The model under review builds one solid part; all positions refer to its coordinate system, in mm. Face numbers are marked on the shaded views. A direction names the side the tool comes from. Round coordinates to 2 decimals unless told otherwise and drop trailing zeros. Order: outer loops, then holes, each group sorted by start corner. A loop starts at its lowest first (then second) coordinate and runs counter-clockwise, first axis right, second up. Notation, with made-up numbers: (64.25, 55) - (82.25, 55) arc R18 cw to (82.25, 78) - close; hole circle Ø9 at (-11.5, -30). An arc over 180 degrees is marked (long way). One line per question, with ' | ' between items. Start each with the question number.
Item 1: Add section C-C on x = 9.25. State the section outline as (y, z) points (3 decimals), and give its area (3 significant figures).
Item 2: Add section A-A on z = -13. State the section outline as (x, y) points (3 decimals).
Item 3: Insertion check: pin 1 Ø12 at (y, z) = (3.5, -1) entering from -X; pin 2 Ø4 at (x, y) = (6.5, 4.5) entering from -Z; pin 3 Ø3.5 at (x, z) = (9.5, -11.5) entering from -Y; pin 4 Ø0.8 at (x, y) = (10, -0.5) entering from -Z. Each pin has a flat end and moves straight along its axis. Give the tip position at first contact, or say it passes through.
Item 4: Add section B-B on y = 4. State the section outline as (x, z) points, and give its area (3 significant figures).
Item 5: For L1, parallel to Z at x = -7, y = 8.5; L2, parallel to Y at x = -10.5, z = -4.5; L3, parallel to Y at x = -16, z = -11.25, list the stretches that pass through material, from the lowest coordinate up. Write a range as [from, to].
Item 6: Tool access review of the marked faces 5, 6, 7, 8 and 9: name each direction out of +Z, -Z, +X, -X, +Y, -Y from which nothing blocks a thin tool from reaching the whole face with its end or side.
Item 7: Add section D-D on z = -22. State the section outline as (x, y) points, and give its area (3 significant figures).
Item 8: Draft analysis for pull direction X (two halves, no side actions). For the marked faces 1, 2, 3 and 4, state which applies: +X half, -X half, draft (parallel to the pull), parting line (faces both ways), or undercut.
from build123d import *

# Parameters (mm, degrees)
F0_W           = 13.375
F0_H           = 2
F1_DEPTH       = 18.25
F2_R           = 1.7808687455
F2_R_2         = 1.7800904517
F3_DEPTH       = 2
F4_W           = 11.3
F4_H           = 30
F5_DEPTH       = 18.25
F6_W           = 26
F6_H           = 6.5
F7_DEPTH       = 30
F9_DEPTH       = 30
F11_DEPTH      = 13
F11_DEPTH_BACK = 13
F12_R          = 1.375
F13_DEPTH      = 4.8
F14_W          = 5.5
F14_H          = 5.5
F15_DEPTH      = 1.5
F16_T1_DEPTH   = 27.75
F16_T3_DEPTH   = 27.75
F16_T5_DEPTH   = 59
F17_SIZE2      = 10.3923048454
F17_SIZE       = 6
F18_T1_DEPTH   = 20.7323463904
F18_T3_DEPTH   = 6.4746360003
F18_T5_DEPTH   = 38.5573463904
F18_T7_DEPTH   = 1.5286731952
F18_T9_DEPTH   = 7.7786731952
F18_T11_DEPTH  = 6.4746360003
F18_T13_DEPTH  = 7.7786731952
F18_T18_DEPTH  = 4.8857735151
F18_T23_DEPTH  = 10.5573463904
F18_T29_DEPTH  = 4.8857735151
F18_T39_DEPTH  = 2.5573463904
F18_T43_DEPTH  = 8.8073463904
F18_T50_DEPTH  = 4.8857735151
F18_T54_DEPTH  = 10.5573463904
F18_T61_DEPTH  = 2.5573463904
F18_T65_DEPTH  = 8.8073463904
F18_T72_DEPTH  = 10.5573463904
F18_T76_DEPTH  = 4.8857735151


# Not quite as in the source:
# - a fillet or chamfer that OpenCascade refuses, or shapes differently, is made with other operations: its cross-section is extruded or revolved along the edge and cut away or added


with BuildPart() as f1:
    # F0 (on Right) → F1 (new body, symmetric)
    with BuildSketch(Plane.YZ):
        with Locations((6.6875, 1)):
            Rectangle(F0_W, F0_H)
    extrude(amount=F1_DEPTH, both=True)

    # F2 (on face) → F3 (cut, through all)
    with BuildSketch(Plane.XY.offset(2)):
        with Locations((6.5276143141, 4)):
            Circle(F2_R)
        with Locations((-6.3883271068, 4)):
            Circle(F2_R_2)
    extrude(amount=-F3_DEPTH, mode=Mode.SUBTRACT)

    # F4 (on Right) → F5 (join, symmetric)
    with BuildSketch(Plane.YZ):
        with Locations((-5.65, -13)):
            Rectangle(F4_W, F4_H)
    extrude(amount=F5_DEPTH, both=True)

    # F6 (on face) → F7 (cut, through all)
    with BuildSketch(Plane(origin=(0, 0, -28), x_dir=(1, 0, 0), z_dir=(0, 0, -1))):
        with Locations((0, 8.05)):
            Rectangle(F6_W, F6_H)
    extrude(amount=-F7_DEPTH, mode=Mode.SUBTRACT)

    # F8 (on face) → F9 (cut, through all)
    with BuildSketch(Plane(origin=(0, 0, -28), x_dir=(1, 0, 0), z_dir=(0, 0, -1))):
        Polygon((6.25, 4.8), (-6.25, 4.8), (-4.25, 2.8), (4.25, 2.8), align=None)
    extrude(amount=-F9_DEPTH, mode=Mode.SUBTRACT)

    # F10 (on Right) → F11 (cut, two sides)
    with BuildSketch(Plane.YZ) as f11_sk:
        Polygon((-4.8, -28), (-2.8, -28), (-4.8, -16), align=None)
    extrude(amount=F11_DEPTH, mode=Mode.SUBTRACT)
    extrude(f11_sk.sketch, amount=-F11_DEPTH_BACK, mode=Mode.SUBTRACT)

    # F12 (on face) → F13 (cut, through all)
    with BuildSketch(Plane.XZ.offset(4.8)):
        with Locations((-9.25, -13)):
            Circle(F12_R)
        with Locations((9.25, -13)):
            Circle(F12_R)
    extrude(amount=-F13_DEPTH, mode=Mode.SUBTRACT)

    # F14 (on face) → F15 (cut)
    with BuildSketch(Plane(origin=(0, 0, 0), x_dir=(-1, 0, 0), z_dir=(0, 1, 0))):
        with Locations((-9.25, -13)):
            Rectangle(F14_W, F14_H)
        with Locations((9.25, -13)):
            Rectangle(F14_W, F14_H)
    extrude(amount=-F15_DEPTH, mode=Mode.SUBTRACT)

    # F16: fillet of radius 4.5 on 3 edges, made by hand

    # F16_s2 → F16_t1 (cut)
    with BuildSketch(Plane.YZ.offset(-29.5)):
        with BuildLine():
            ThreePointArc((-11.3, -23.5), (-9.9819805153, -26.6819805153), (-6.8, -28))
            Line((-6.8, -28), (-11.3, -28))
            Line((-11.3, -28), (-11.3, -23.5))
        make_face()
    extrude(amount=F16_T1_DEPTH, mode=Mode.SUBTRACT)

    # F16_s4 → F16_t3 (cut)
    with BuildSketch(Plane.YZ.offset(1.75)):
        with BuildLine():
            ThreePointArc((-6.8, -28), (-9.9819805153, -26.6819805153), (-11.3, -23.5))
            Line((-11.3, -23.5), (-11.3, -28))
            Line((-11.3, -28), (-6.8, -28))
        make_face()
    extrude(amount=F16_T3_DEPTH, mode=Mode.SUBTRACT)

    # F16_s6 → F16_t5 (cut)
    with BuildSketch(Plane.YZ.offset(-29.5)):
        with BuildLine():
            ThreePointArc((-4.5, -28), (-1.3180194847, -26.6819805153), (0, -23.5))
            Line((0, -23.5), (0, -28))
            Line((0, -28), (-4.5, -28))
        make_face()
    extrude(amount=F16_T5_DEPTH, mode=Mode.SUBTRACT)

    # F17
    f17_edges = [f1.edges().sort_by_distance(p)[0] for p in [
        (-15.625, -11.3, 2),
        (15.625, -11.3, 2),
    ]]
    f17_side = f1.faces().sort_by_distance((-0.00209, 3.324537, 2))[0]
    chamfer(f17_edges, length=F17_SIZE, length2=F17_SIZE2, reference=f17_side)

    # F18: chamfer of 0.4 on 14 edges, made by hand

    # F18_s2 → F18_t1 (cut)
    with BuildSketch(Plane.XZ.offset(-14.4036731952)):
        Polygon((-18.25, 1.6), (-17.85, 2), (-18.25, 2), align=None)
        Polygon((17.85, 2), (18.25, 1.6), (18.25, 2), align=None)
    extrude(amount=F18_T1_DEPTH, mode=Mode.SUBTRACT)

    # F18_s4 → F18_t3 (cut)
    with BuildSketch(Plane.YZ.offset(-18.8623180002)):
        Polygon((-5.4154700538, 1.8), (-5.0690598923, 2), (-5.3, 2), align=None)
    extrude(amount=F18_T3_DEPTH, mode=Mode.SUBTRACT)

    # F18_s6 → F18_t5 (cut)
    with BuildSketch(Plane.YZ.offset(-19.2786731952)):
        Polygon((12.975, 2), (13.375, 1.6), (13.375, 2), align=None)
    extrude(amount=F18_T5_DEPTH, mode=Mode.SUBTRACT)

    # F18_s8 → F18_t7 (cut)
    with BuildSketch(Plane.XZ.offset(4.8)):
        Polygon((-13.4, 2), (-13, 1.6), (-13, 2), align=None)
        Polygon((13.4, 2), (13, 1.6), (13, 2), align=None)
    extrude(amount=F18_T7_DEPTH, mode=Mode.SUBTRACT)

    # F18_s10 → F18_t9 (cut)
    with BuildSketch(Plane.YZ.offset(-13)):
        Polygon((-4.4, 2), (-4.8, 1.6), (-4.8, 2), align=None)
    extrude(amount=F18_T9_DEPTH, mode=Mode.SUBTRACT)

    # F18_s12 → F18_t11 (cut)
    with BuildSketch(Plane.YZ.offset(12.3876819998)):
        Polygon((-5.0690598923, 2), (-5.4154700538, 1.8), (-5.3, 2), align=None)
    extrude(amount=F18_T11_DEPTH, mode=Mode.SUBTRACT)

    # F18_s14 → F18_t13 (cut)
    with BuildSketch(Plane.YZ.offset(5.2213268048)):
        Polygon((-4.4, 2), (-4.8, 1.6), (-4.8, 2), align=None)
    extrude(amount=F18_T13_DEPTH, mode=Mode.SUBTRACT)


with BuildPart() as f18_tool16:
    # F18_s17 → F18_t18 (new body)
    with BuildSketch(Plane(origin=(-6.2523817919, -6.2523817919, 0), x_dir=(0, 0, 1), z_dir=(0.7071067812, 0.7071067812, 0))):
        Polygon((2, -1.4253048327), (1.6, -1.0253048327), (2, -1.0253048327), align=None)
    extrude(amount=F18_T18_DEPTH)

    split(bisect_by=Plane.XZ.offset(2.8), keep=Keep.TOP)


with BuildPart() as f1_1:
    add(f1.part)

    # F18_t15: cut F18_tool16
    add(f18_tool16.part, mode=Mode.SUBTRACT)


with BuildPart() as f18_tool21:
    # F18_s22 → F18_t23 (new body)
    with BuildSketch(Plane.YZ.offset(-5.2786731952)):
        Polygon((-2.4, 2), (-2.8, 1.6), (-2.8, 2), align=None)
    extrude(amount=F18_T23_DEPTH)

    split(bisect_by=Plane(origin=(-0.725, 0.725, 0), x_dir=(0, 0, 1), z_dir=(0.7071067812, -0.7071067812, 0)), keep=Keep.TOP)

    split(bisect_by=Plane(origin=(0.725, 0.725, 0), x_dir=(0, 0, 1), z_dir=(-0.7071067812, -0.7071067812, 0)), keep=Keep.TOP)


with BuildPart() as f1_2:
    add(f1_1.part)

    # F18_t20: cut F18_tool21
    add(f18_tool21.part, mode=Mode.SUBTRACT)


with BuildPart() as f18_tool27:
    # F18_s28 → F18_t29 (new body)
    with BuildSketch(Plane(origin=(2.7976182081, -2.7976182081, 0), x_dir=(0, 0, 1), z_dir=(0.7071067812, -0.7071067812, 0))):
        Polygon((2, -1.4253048327), (1.6, -1.0253048327), (2, -1.0253048327), align=None)
    extrude(amount=F18_T29_DEPTH)

    split(bisect_by=Plane.XZ.offset(2.8), keep=Keep.TOP)


with BuildPart() as f1_3:
    add(f1_2.part)

    # F18_t26: cut F18_tool27
    add(f18_tool27.part, mode=Mode.SUBTRACT)

    # F18_s31 → F18_t32 (revolve, cut)
    with BuildSketch(Plane.XZ.offset(-4)):
        Polygon((-4.2082366551, 2), (-4.6082366551, 1.6), (-4.6082366551, 2), align=None)
    revolve(axis=Axis((-6.3883271068, 4, 2), (0, 0, 1)), mode=Mode.SUBTRACT)

    # F18_s33 → F18_t34 (revolve, cut)
    with BuildSketch(Plane.XZ.offset(-4)):
        Polygon((8.7084830596, 2), (8.3084830596, 1.6), (8.3084830596, 2), align=None)
    revolve(axis=Axis((6.5276143141, 4, 2), (0, 0, 1)), mode=Mode.SUBTRACT)


with BuildPart() as f18_tool37:
    # F18_s38 → F18_t39 (new body)
    with BuildSketch(Plane.XZ.offset(6.3286731952)):
        Polygon((-13.4, 2), (-13, 1.6), (-13, 2), align=None)
    extrude(amount=-F18_T39_DEPTH)

    split(bisect_by=Plane.XZ.offset(4.8), keep=Keep.BOTTOM)


with BuildPart() as f18_tool41:
    # F18_s42 → F18_t43 (new body)
    with BuildSketch(Plane.YZ.offset(-14.0286731952)):
        Polygon((-4.4, 2), (-4.8, 1.6), (-4.8, 2), align=None)
    extrude(amount=F18_T43_DEPTH)

    split(bisect_by=Plane.YZ.offset(-13), keep=Keep.BOTTOM)


with BuildPart() as f18_tool37_1:
    add(f18_tool37.part)

    # F18_t45: intersect F18_tool41
    add(f18_tool41.part, mode=Mode.INTERSECT)


with BuildPart() as f1_4:
    add(f1_3.part)

    # F18_t35: cut F18_tool37
    add(f18_tool37_1.part, mode=Mode.SUBTRACT)


with BuildPart() as f18_tool48:
    # F18_s49 → F18_t50 (new body)
    with BuildSketch(Plane(origin=(-6.2523817919, -6.2523817919, 0), x_dir=(0, 0, 1), z_dir=(0.7071067812, 0.7071067812, 0))):
        Polygon((2, -1.4253048327), (1.6, -1.0253048327), (2, -1.0253048327), align=None)
    extrude(amount=F18_T50_DEPTH)

    split(bisect_by=Plane.XZ.offset(2.8), keep=Keep.BOTTOM)


with BuildPart() as f18_tool52:
    # F18_s53 → F18_t54 (new body)
    with BuildSketch(Plane.YZ.offset(-5.2786731952)):
        Polygon((-2.4, 2), (-2.8, 1.6), (-2.8, 2), align=None)
    extrude(amount=F18_T54_DEPTH)

    split(bisect_by=Plane(origin=(-0.725, 0.725, 0), x_dir=(0, 0, 1), z_dir=(-0.7071067812, 0.7071067812, 0)), keep=Keep.TOP)


with BuildPart() as f18_tool48_1:
    add(f18_tool48.part)

    # F18_t56: intersect F18_tool52
    add(f18_tool52.part, mode=Mode.INTERSECT)


with BuildPart() as f1_5:
    add(f1_4.part)

    # F18_t46: cut F18_tool48
    add(f18_tool48_1.part, mode=Mode.SUBTRACT)


with BuildPart() as f18_tool59:
    # F18_s60 → F18_t61 (new body)
    with BuildSketch(Plane.XZ.offset(3.7713268048)):
        Polygon((13.4, 2), (13, 1.6), (13, 2), align=None)
    extrude(amount=F18_T61_DEPTH)

    split(bisect_by=Plane.XZ.offset(4.8), keep=Keep.BOTTOM)


with BuildPart() as f18_tool63:
    # F18_s64 → F18_t65 (new body)
    with BuildSketch(Plane.YZ.offset(5.2213268048)):
        Polygon((-4.4, 2), (-4.8, 1.6), (-4.8, 2), align=None)
    extrude(amount=F18_T65_DEPTH)

    split(bisect_by=Plane.YZ.offset(13), keep=Keep.TOP)


with BuildPart() as f18_tool59_1:
    add(f18_tool59.part)

    # F18_t67: intersect F18_tool63
    add(f18_tool63.part, mode=Mode.INTERSECT)


with BuildPart() as f1_6:
    add(f1_5.part)

    # F18_t57: cut F18_tool59
    add(f18_tool59_1.part, mode=Mode.SUBTRACT)


with BuildPart() as f18_tool70:
    # F18_s71 → F18_t72 (new body)
    with BuildSketch(Plane.YZ.offset(-5.2786731952)):
        Polygon((-2.4, 2), (-2.8, 1.6), (-2.8, 2), align=None)
    extrude(amount=F18_T72_DEPTH)

    split(bisect_by=Plane(origin=(0.725, 0.725, 0), x_dir=(0, 0, 1), z_dir=(0.7071067812, 0.7071067812, 0)), keep=Keep.TOP)


with BuildPart() as f18_tool74:
    # F18_s75 → F18_t76 (new body)
    with BuildSketch(Plane(origin=(2.7976182081, -2.7976182081, 0), x_dir=(0, 0, 1), z_dir=(0.7071067812, -0.7071067812, 0))):
        Polygon((2, -1.4253048327), (1.6, -1.0253048327), (2, -1.0253048327), align=None)
    extrude(amount=F18_T76_DEPTH)

    split(bisect_by=Plane.XZ.offset(2.8), keep=Keep.BOTTOM)


with BuildPart() as f18_tool70_1:
    add(f18_tool70.part)

    # F18_t78: intersect F18_tool74
    add(f18_tool74.part, mode=Mode.INTERSECT)


with BuildPart() as f1_7:
    add(f1_6.part)

    # F18_t68: cut F18_tool70
    add(f18_tool70_1.part, mode=Mode.SUBTRACT)


solid = f1_7.part
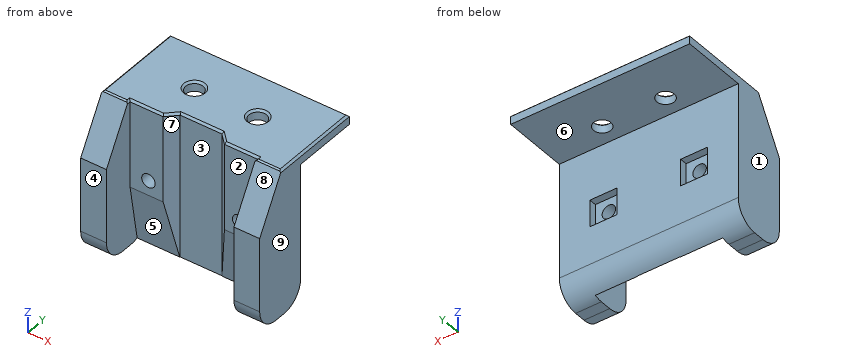
Determined:
1) outline: (-4.8, -16) - (-2.852, -27.687) arc R4.5 ccw to (0, -23.5) - (0, -15.75) - (-1.5, -15.75) - (-1.5, -14.375) - (-4.8, -14.375) - close; (-4.8, -11.625) - (-1.5, -11.625) - (-1.5, -10.25) - (0, -10.25) - (0, 0) - (13.375, 0) - (13.375, 1.6) - (12.975, 2) - (-4.4, 2) - (-4.8, 1.6) - close | area: 137 mm2
2) outline: (-18.25, -11.3) - (-13, -11.3) - (-13, -4.8) - (-10.625, -4.8) - (-10.625, -1.5) - (-12, -1.5) - (-12, 0) - (-18.25, 0) - close; (-7.875, -4.8) - (-6.25, -4.8) - (-4.25, -2.8) - (4.25, -2.8) - (6.25, -4.8) - (7.875, -4.8) - (7.875, -1.5) - (6.5, -1.5) - (6.5, 0) - (-6.5, 0) - (-6.5, -1.5) - (-7.875, -1.5) - close; (10.625, -4.8) - (13, -4.8) - (13, -11.3) - (18.25, -11.3) - (18.25, 0) - (12, 0) - (12, -1.5) - (10.625, -1.5) - close
3) pin 1: x = -18.25 | pin 2: z = 0 | pin 3: y = -4.8 | pin 4: z = -26.2
4) outline: (-18.25, 0) - (-8.17, 0) - (-8.17, 1.6) - (-8.57, 2) - (-17.85, 2) - (-18.25, 1.6) - close; (-4.61, 0) - (4.75, 0) - (4.75, 1.6) - (4.35, 2) - (-4.21, 2) - (-4.61, 1.6) - close; (8.31, 0) - (18.25, 0) - (18.25, 1.6) - (17.85, 2) - (8.71, 2) - (8.31, 1.6) - close | area: 58.3 mm2
5) L1: [0, 2] | L2: [-4.8, 0] | L3: [-11.3, 0]
6) face 5: -Z, -Y | face 6: -Z, +X, -X, +Y | face 7: +Z, -Z, -Y | face 8: +Z, +X, -X, -Y | face 9: +Z, -Z, +X, +Y, -Y
7) outline: (-18.25, -11.3) - (-13, -11.3) - (-13, -3.8) - (-5.25, -3.8) - (-4.25, -2.8) - (4.25, -2.8) - (5.25, -3.8) - (13, -3.8) - (13, -11.3) - (18.25, -11.3) - (18.25, 0) - (-18.25, 0) - close | area: 208 mm2
8) face 1: -X half | face 2: undercut | face 3: undercut | face 4: draft
